Geometry check sheet. Reference: the model listing, model coordinates, mm. A direction names the side the tool comes from. Coordinates: 2 decimals unless noted, no trailing zeros. Write each loop counter-clockwise with the first axis right and the second up, starting at its lowest first coordinate (ties: lowest second). Pieces come first, ordered by that corner, then holes.
from build123d import *

# Parameters (mm, degrees)
BOSS_EXTRUDE1_DEPTH   = 2.54
SKETCH1_4_R           = 7.325
SKETCH1_4_R_2         = 4.15
SKETCH1_4_R_3         = 7.175
BOSS_EXTRUDE2_DEPTH   = 25.4
F_8_CLEARANCE_HOLE2_D = 4.4958
LPATTERN1_COUNT       = 2
LPATTERN1_PITCH       = 116.586
LPATTERN1_COUNT_DIR2  = 2
LPATTERN1_PITCH_DIR2  = 69.85


with BuildPart() as part:
    # Sketch1 → Boss-Extrude1 (new body)
    with BuildSketch(Plane(origin=(0, 0, 0), x_dir=(1, 0, 0), z_dir=(0, 1, 0))):
        with BuildLine():
            ThreePointArc((8.209871939, -17.190128061), (15.555896424, -34.925), (8.209871939, -52.659871939))
            ThreePointArc((8.209871939, -52.659871939), (0, -57.15), (-8.209871939, -52.659871939))
            ThreePointArc((-8.209871939, -52.659871939), (-17.190128061, -52.659871939), (-17.190128061, -61.640128061))
            ThreePointArc((-17.190128061, -61.640128061), (-13.499098781, -66.567297756), (-11.341832503, -72.333310292))
            ThreePointArc((-11.341832503, -72.333310292), (0, -81.460512242), (11.341832503, -72.333310292))
            ThreePointArc((11.341832503, -72.333310292), (13.499098781, -66.567297756), (17.190128061, -61.640128061))
            ThreePointArc((17.190128061, -61.640128061), (58.293, -44.614761051), (99.395871939, -61.640128061))
            ThreePointArc((99.395871939, -61.640128061), (103.086901219, -66.567297756), (105.244167497, -72.333310292))
            ThreePointArc((105.244167497, -72.333310292), (116.586, -81.460512242), (127.927832503, -72.333310292))
            ThreePointArc((127.927832503, -72.333310292), (130.085098781, -66.567297756), (133.776128061, -61.640128061))
            ThreePointArc((133.776128061, -61.640128061), (133.776128061, -52.659871939), (124.795871939, -52.659871939))
            ThreePointArc((124.795871939, -52.659871939), (116.586, -57.15), (108.376128061, -52.659871939))
            ThreePointArc((108.376128061, -52.659871939), (101.030103576, -34.925), (108.376128061, -17.190128061))
            ThreePointArc((108.376128061, -17.190128061), (116.586, -12.7), (124.795871939, -17.190128061))
            ThreePointArc((124.795871939, -17.190128061), (133.776128061, -17.190128061), (133.776128061, -8.209871939))
            ThreePointArc((133.776128061, -8.209871939), (130.085098781, -3.282702244), (127.927832503, 2.483310292))
            ThreePointArc((127.927832503, 2.483310292), (116.825136798, 11.608049281), (105.356064016, 2.948310079))
            ThreePointArc((105.356064016, 2.948310079), (103.204339104, -3.073259016), (99.395871939, -8.209871939))
            ThreePointArc((99.395871939, -8.209871939), (58.293, -25.235238949), (17.190128061, -8.209871939))
            ThreePointArc((17.190128061, -8.209871939), (13.381660896, -3.073259016), (11.229935984, 2.948310079))
            ThreePointArc((11.229935984, 2.948310079), (-0.239136798, 11.608049281), (-11.341832503, 2.483310292))
            ThreePointArc((-11.341832503, 2.483310292), (-13.499098781, -3.282702244), (-17.190128061, -8.209871939))
            ThreePointArc((-17.190128061, -8.209871939), (-17.190128061, -17.190128061), (-8.209871939, -17.190128061))
            ThreePointArc((-8.209871939, -17.190128061), (0, -12.7), (8.209871939, -17.190128061))
        make_face()
    extrude(amount=BOSS_EXTRUDE1_DEPTH)

    # Sketch1_4 → Boss-Extrude2 (add)
    # profile 1 of 4: a face of its own
    with BuildSketch(Plane(origin=(0, 0, 0), x_dir=(1, 0, 0), z_dir=(0, 1, 0))):
        with Locations(Location((0, 0, 0), (0, 0, 270))):
            Circle(SKETCH1_4_R)
        with Locations(Location((0, 0, 0), (0, 0, 270))):
            Circle(SKETCH1_4_R_2, mode=Mode.SUBTRACT)
    # profile 2 of 4: a face of its own
    with BuildSketch(Plane(origin=(0, 0, 0), x_dir=(1, 0, 0), z_dir=(0, 1, 0))):
        with Locations(Location((116.586, 0, 0), (0, 0, 270))):
            Circle(SKETCH1_4_R_3)
        with Locations(Location((116.586, 0, 0), (0, 0, 270))):
            Circle(SKETCH1_4_R_2, mode=Mode.SUBTRACT)
    # profile 3 of 4: a face of its own
    with BuildSketch(Plane(origin=(0, 0, 0), x_dir=(1, 0, 0), z_dir=(0, 1, 0))):
        with Locations(Location((0, -69.85, 0), (0, 0, 270))):
            Circle(SKETCH1_4_R_3)
        with Locations(Location((0, -69.85, 0), (0, 0, 270))):
            Circle(SKETCH1_4_R_2, mode=Mode.SUBTRACT)
    # profile 4 of 4: a face of its own
    with BuildSketch(Plane(origin=(0, 0, 0), x_dir=(1, 0, 0), z_dir=(0, 1, 0))):
        with Locations(Location((116.586, -69.85, 0), (0, 0, 270))):
            Circle(SKETCH1_4_R_3)
        with Locations(Location((116.586, -69.85, 0), (0, 0, 270))):
            Circle(SKETCH1_4_R_2, mode=Mode.SUBTRACT)
    extrude(amount=BOSS_EXTRUDE2_DEPTH)

    # 8 Clearance Hole2 (through all)
    with Locations(Plane(origin=(0, 2.54, 0), x_dir=(1, 0, 0), z_dir=(0, 1, 0))):
        with Locations((129.286, -12.7), (129.286, -57.15), (-12.7, -57.15), (-12.7, -12.7)):
            Hole(F_8_CLEARANCE_HOLE2_D / 2)

    # Sketch8 → Revolve1 (revolve)
    with BuildSketch(Plane(origin=(0, 0, 0), x_dir=(0, 0, -1), z_dir=(1, 0, 0))):
        Polygon((10.856911267, 2.54), (7.046911267, 21.59), (7.046911267, 2.54), align=None)
    revolve1 = revolve(axis=Axis((0, 0, 0), (0, 1, 0)))

    # LPattern1: Revolve1 2 × 2
    with Locations(*[(i * LPATTERN1_PITCH, 0, j * LPATTERN1_PITCH_DIR2) for i in range(LPATTERN1_COUNT) for j in range(LPATTERN1_COUNT_DIR2) if (i, j) != (0, 0)]):
        add(revolve1)


solid = part.part
1. Sectioned sample at B-B, the plane x = 0. Record the boundary of the cut face in (y, z) (3 decimals), and give its area (3 significant figures).
Computed values:
outline: (0, -11.611) - (2.54, -11.611) - (2.54, -10.857) - (20.2, -7.325) - (25.4, -7.325) - (25.4, -4.15) - (2.54, -4.15) - (2.54, 4.15) - (25.4, 4.15) - (25.4, 7.325) - (20.2, 7.325) - (2.54, 10.857) - (2.54, 12.7) - (0, 12.7) - close; (0, 57.15) - (2.54, 57.15) - (2.54, 58.993) - (20.95, 62.675) - (25.4, 62.675) - (25.4, 65.7) - (2.54, 65.7) - (2.54, 74) - (25.4, 74) - (25.4, 77.025) - (20.95, 77.025) - (2.54, 80.707) - (2.54, 81.461) - (0, 81.461) - close
area: 537 mm2
2. Draft check along Z on faces 1 (the cylindrical face through (-13.46, 1.25, 3.21)), 2 (the cylindrical face through (-2.53, 13.81, -3.29)), 3 (the cylindrical face through (103.045, 1.252, 66.492)). Enter one of: released by +Z, released by -Z, zero draft, split by the parting line, or undercut.
Computed values:
face 1: released by -Z
face 2: undercut
face 3: released by +Z
3. Thickness scan on line 1 along Z through (x, y) = (0, 20.75) (3 decimals); line 2 along Z through (x, y) = (3.5, 20.75); line 3 along X through (y, z) = (11.75, 69.85). Record the ranges inside material, lowest first.
Computed values:
line 1: z = -7.325 to -4.15, 4.15 to 7.325, 62.635 to 65.7, 74 to 77.065
line 2: z = -6.43 to -2.23, 2.23 to 6.43, 63.54 to 67.62, 72.08 to 76.16
line 3: x = -9.01 to -4.15, 4.15 to 9.01, 107.57 to 112.44, 120.74 to 125.6
4. Gauge pin test, flat ends, axial feed: pin 1 Ø5 at (x, z) = (116.586, 69.85) entering from +Y; pin 2 Ø10 at (y, z) = (17.5, 67.5) entering from -X; pin 3 Ø11 at (x, z) = (0, 69.85) entering from +Y; pin 4 Ø3.5 at (x, z) = (-12.7, 57.15) entering from -Y. Record the tip position at first contact, or that the pin passes through.
Computed values:
pin 1: stops at y = 2.54
pin 2: stops at x = -8.78
pin 3: stops at y = 25.4
pin 4: passes through
5. Access from +Z, -Z, +X, -X, +Y, -Y to the whole of each face (thin tool, end or side, straight path). Record for faces 4 (the cylindrical face through (103.25, 1.25, 2.99)), 5 (the cylindrical face through (116.4, 1.3, 12.7)), 6 (the cylindrical face through (1.247, 13.81, 73.808)).
Computed values:
face 4: -Z, +Y, -Y
face 5: +Y, -Y
face 6: +Y
6. Sectioned sample at A-A, the plane y = 10.75. Record the boundary of the cut face in (x, z), and give its area (3 significant figures).
Computed values:
outline: circle Ø18.43 at (0, 0); circle Ø18.43 at (0, 69.85); circle Ø18.43 at (116.59, 0); circle Ø18.43 at (116.59, 69.85); hole circle Ø8.3 at (0, 0); hole circle Ø8.3 at (0, 69.85); hole circle Ø8.3 at (116.59, 0); hole circle Ø8.3 at (116.59, 69.85)
area: 851 mm2
7. Sectioned sample at D-D, the plane y = 23.5. Record the boundary of the cut face in (x, z) (3 decimals), and give its area (3 significant figures).
Computed values:
outline: circle Ø14.65 at (0, 0); circle Ø14.35 at (0, 69.85); circle Ø14.35 at (116.586, 0); circle Ø14.35 at (116.586, 69.85); hole circle Ø8.3 at (0, 0); hole circle Ø8.3 at (0, 69.85); hole circle Ø8.3 at (116.586, 0); hole circle Ø8.3 at (116.586, 69.85)
area: 437 mm2
8. Sectioned sample at C-C, the plane z = 0. Record the boundary of the cut face in (x, y) (3 decimals).
Computed values:
outline: (-12.043, 0) - (12.033, 0) - (12.033, 2.54) - (10.857, 2.54) - (7.325, 20.2) - (7.325, 25.4) - (4.15, 25.4) - (4.15, 2.54) - (-4.15, 2.54) - (-4.15, 25.4) - (-7.325, 25.4) - (-7.325, 20.2) - (-10.857, 2.54) - (-12.043, 2.54) - close; (104.553, 0) - (128.629, 0) - (128.629, 2.54) - (127.443, 2.54) - (123.761, 20.95) - (123.761, 25.4) - (120.736, 25.4) - (120.736, 2.54) - (112.436, 2.54) - (112.436, 25.4) - (109.411, 25.4) - (109.411, 20.95) - (105.729, 2.54) - (104.553, 2.54) - close
